```python
from build123d import *

# Parameters (mm, degrees)
DODANIE_WYCI_GNI_CIE1_DEPTH       = 25
DODANIE_WYCI_GNI_CIE2_DEPTH       = 5
WYCI_GNI_CIE_CIENKA_CIANKA1_REACH = 150.354
ZAOKR_GLENIE1_R                   = 10
ZAOKR_GLENIE2_R                   = 10
ZAOKR_GLENIE3_R                   = 10
ZAOKR_GLENIE4_R                   = 10


with BuildPart() as part:
    # Szkic1 → Dodanie-wyci_gni_cie1 (new body)
    with BuildSketch(Plane(origin=(0, 0, 0), x_dir=(1, 0, 0), z_dir=(0, 1, 0))):
        with BuildLine():
            Line((0, 20), (0, 15))
            ThreePointArc((0, 15), (-15, 0), (0, -15))
            Line((0, -15), (0, -20))
            ThreePointArc((0, -20), (-20, 0), (0, 20))
        make_face()
    extrude(amount=DODANIE_WYCI_GNI_CIE1_DEPTH)

    # Szkic2 → Dodanie-wyci_gni_cie2 (add)
    with BuildSketch(Plane(origin=(0, 0, 0), x_dir=(1, 0, 0), z_dir=(0, 1, 0))):
        with BuildLine():
            Line((0, 20), (0, 72))
            Line((0, 72), (-40, 72))
            Line((-40, 72), (-40, 44.72135955))
            ThreePointArc((-40, 44.72135955), (-56.050341538, -21.409325386), (0, -60))
            Line((0, -60), (0, -20))
            ThreePointArc((0, -20), (-20, 0), (0, 20))
        make_face()
    extrude(amount=DODANIE_WYCI_GNI_CIE2_DEPTH)


with BuildPart() as body_2:
    # Lustro3: mirrored copy
    add(part.part.mirror(Plane.ZX.offset(-45)))

    # Szkic3 → Wyci_gni_cie-cienka _cianka1 (add, up to next)
    with BuildSketch(Plane(origin=(0, 0, 0), x_dir=(1, 0, 0), z_dir=(0, 1, 0)), mode=Mode.PRIVATE) as wyci_gni_cie_cienka_cianka1_sk1:
        with BuildLine():
            Line((-40, 72), (-40, 44.72135955))
            ThreePointArc((-40, 44.72135955), (-56.050341538, -21.409325386), (0, -60))
            Line((0, -60), (0, -55))
            ThreePointArc((0, -55), (-51.76124215, -18.594994247), (-35, 42.426406871))
            Line((-35, 42.426406871), (-35, 72))
            Line((-35, 72), (-40, 72))
        make_face()
    wyci_gni_cie_cienka_cianka1_tool1 = extrude(wyci_gni_cie_cienka_cianka1_sk1.sketch, amount=-WYCI_GNI_CIE_CIENKA_CIANKA1_REACH, mode=Mode.PRIVATE) - body_2.part

    add(part.part)  # Wyci_gni_cie-cienka _cianka1 merges part
    add(wyci_gni_cie_cienka_cianka1_tool1.solids().sort_by_distance((-36.449966, 0, -57.213203))[0])

    # Zaokr_glenie1
    zaokr_glenie1_edges = [body_2.edges().sort_by_distance(p)[0] for p in [
        (-40, 5, -58.360679775),
    ]]
    fillet(zaokr_glenie1_edges, radius=ZAOKR_GLENIE1_R)

    # Zaokr_glenie2
    zaokr_glenie2_edges = [body_2.edges().sort_by_distance(p)[0] for p in [
        (-40, -95, -58.360679775),
    ]]
    fillet(zaokr_glenie2_edges, radius=ZAOKR_GLENIE2_R)

    # Zaokr_glenie3
    zaokr_glenie3_edges = [body_2.edges().sort_by_distance(p)[0] for p in [
        (-35, 0, -57.213203436),
    ]]
    fillet(zaokr_glenie3_edges, radius=ZAOKR_GLENIE3_R)

    # Zaokr_glenie4
    zaokr_glenie4_edges = [body_2.edges().sort_by_distance(p)[0] for p in [
        (-35, -90, -57.213203436),
    ]]
    fillet(zaokr_glenie4_edges, radius=ZAOKR_GLENIE4_R)


solid = body_2.part
```
Can you work these out from the model? Positions are in its coordinate system, mm. A direction names the side the tool comes from. Coordinates: 2 decimals unless noted, no trailing zeros. Loops run counter-clockwise (first coordinate to the right, second up) from the corner with the lowest first, then second, coordinate; pieces in that order, holes last. Notation, with made-up numbers: (79, 86) -> (123, 86) arc R22 cw to (123, 97) -> close; hole circle Ø9 at (-36, -33.5). An arc over 180 degrees is marked (long way). Answer as a JSON object with one key per item and string values.
1) Imagine slicing it at A-A (y = -19.5). Please give me the cut outline in (x, z), then the cut area to 3 significant figures.
Results:
{"outline": "(-40, -72) -> (-35, -72) -> (-35, -42.43) arc R55 cw to (0, 55) -> (0, 60) arc R60 ccw to (-40, -44.72) -> close", "area": "841 mm^2"}
2) Imagine slicing it at B-B (z = 0). Please give me the cut outline in (x, y), then the cut area to 3 significant figures.
Results:
{"outline": "(-60, -95) -> (-20, -95) -> (-20, -115) -> (-15, -115) -> (-15, -90) -> (-55, -90) -> (-55, 0) -> (-15, 0) -> (-15, 25) -> (-20, 25) -> (-20, 5) -> (-60, 5) -> close", "area": "1,100 mm^2"}
3) If I drill on line 1 (Y direction, x = -16, z = 33.5); line 2 (Z direction, x = -48, y = -5); line 3 (Z direction, x = -50.5, y = -25.5), over which ranges is the centre line in solid material (lowest first)?
Results:
{"line 1": "y = -95 to -90, 0 to 5", "line 2": "z = -36 to -26.85, 26.85 to 36", "line 3": "z = -32.4 to -21.79, 21.79 to 32.4"}
4) For faces 5 (the face through (-31.99, -87.15, -57.01)), 6 (the face through (-22, 0, -9)), 7 (the face through (-20, -105, 0)), 8 (the face through (-40, -44, -59)), 9 (the face through (-37.15, 1.99, -58.17)), which set-ups out of +Z, -Z, +X, -X, +Y, -Y let a thin tool reach every point of the face, with its end or its side?
Results:
{"face 5": "-Z, +X", "face 6": "+X", "face 7": "-X, -Y", "face 8": "-Z, -X, +Y, -Y", "face 9": "-Z, -X, +Y"}
5) Imagine slicing it at D-D (y = 16.5). Please give me the cut outline in (x, z).
Results:
{"outline": "(0, -20) -> (0, -15) arc R15 cw to (0, 15) -> (0, 20) arc R20 ccw to start"}
6) Thinking about a two-plate mould opening in Y: for faces 1 (the face through (-22, -90, -9)), 2 (the face through (-15.1, 25, 1.4)), 3 (the face through (-36, -45, -72)), 4 (the face through (-37.15, -91.99, -58.17)), which applies, pulls with the +Y half, pulls with the -Y half, needs draft (parallel to the pull), parting line crosses it, or undercut?
Results:
{"face 1": "undercut", "face 2": "pulls with the +Y half", "face 3": "needs draft", "face 4": "pulls with the -Y half"}
7) For P1, Ø6, axis at x = -45, z = -43.5, coming from the -Y side; P2, Ø1.5, axis at y = -11, z = -23, coming from the -X side; P3, Ø10, axis at x = -10.5, y = -16, coming from the -Z side, each with a flat end and sliding along its axis, tell me the tip position at first contact or that it passes through.
Results:
{"P1": "stops at y = -95", "P2": "stops at x = -55.72", "P3": "stops at z = 52.77"}
8) Imagine slicing it at C-C (z = 47). Please give me the cut outline in (x, y), then the cut area to 3 significant figures.
Results:
{"outline": "(-37.3, -95) -> (0, -95) -> (0, -90) -> (-28.57, -90) -> (-28.57, 0) -> (0, 0) -> (0, 5) -> (-37.3, 5) -> close", "area": "1,160 mm^2"}
